from build123d import *

# Parameters (mm, degrees)
ESQUISSE1_R        = 2
BOSS_EXTRU_1_DEPTH = 3


with BuildPart() as part:
    # Esquisse1 → Boss.-Extru.1 (new body)
    with BuildSketch(Plane.XY):
        with BuildLine():
            Line((-5.5, 15), (-25.980762114, 15))
            ThreePointArc((-25.980762114, 15), (-30, 0), (-25.980762114, -15))
            Line((-25.980762114, -15), (25.980762114, -15))
            ThreePointArc((25.980762114, -15), (30, 0), (25.980762114, 15))
            Line((25.980762114, 15), (5.5, 15))
            Line((5.5, 15), (5.5, 4.330127019))
            ThreePointArc((5.5, 4.330127019), (0, -7), (-5.5, 4.330127019))
            Line((-5.5, 4.330127019), (-5.5, 15))
        make_face()
        with Locations((-25, 0)):
            Circle(ESQUISSE1_R, mode=Mode.SUBTRACT)
        with Locations((25, 0)):
            Circle(ESQUISSE1_R, mode=Mode.SUBTRACT)
    extrude(amount=BOSS_EXTRU_1_DEPTH)


solid = part.part
Could you check a few things on this model? Use its own coordinates, in mm. A direction names the side the tool comes from. Give positions to 0.01 mm unless a question says otherwise; leave off trailing zeros. Order: outer loops, then holes, each group sorted by start corner. A loop starts at its lowest first (then second) coordinate and runs counter-clockwise, first axis right, second up.
1. For faces 1 (the flat face through (6, 4, 0)), 2 (the flat face through (5.5, 10, 1)), which set-ups out of +Z, -Z, +X, -X, +Y, -Y let a thin tool reach every point of the face, with its end or its side?
2. Suppose I cut it at B-B (y = 0). List the corners of the cut face in (x, z) for me, plus the area to 3 significant figures.
3. Suppose I cut it at A-A (x = -25). List the corners of the cut face in (y, z) for me, plus the area to 3 significant figures.
4. Will this pin go through, and if not, where does the flat tip stop? P1, Ø0.9, axis at y = 8.5, z = 2, coming from the +X side.
5. I need wall thicknesses on L1, parallel to Y at x = 25, z = 2.4; L2, parallel to X at y = 8.5, z = 1.9; L3, parallel to X at y = -6, z = 1.35. Which ranges of each line are inside material? Lowest first, please.
6. We'd pull the mould along Y, two halves only. Please class faces 3 (the cylindrical face through (-27, 0, 1)), 4 (the flat face through (-16, 15, 1)), 5 (the flat face through (0, -15, 1)), 6 (the cylindrical face through (-30, 0, 1)): pulls with the +Y half, pulls with the -Y half, needs draft (parallel to the pull), parting line crosses it, or undercut.
7. Suppose I cut it at D-D (y = 7.75). List the corners of the cut face in (x, z) for me.
8. Suppose I cut it at C-C (z = 0.9). List the corners of the cut face in (x, y) for me.
Solved:
1. face 1: -Z, +X, -X, +Y, -Y
1. face 2: +Z, -Z, +Y
2. outline: (-30, 0) - (-27, 0) - (-27, 3) - (-30, 3) - close; (-23, 0) - (-7, 0) - (-7, 3) - (-23, 3) - close; (7, 0) - (23, 0) - (23, 3) - (7, 3) - close; (27, 0) - (30, 0) - (30, 3) - (27, 3) - close
2. area: 114 mm2
3. outline: (-15, 0) - (-2, 0) - (-2, 3) - (-15, 3) - close; (2, 0) - (15, 0) - (15, 3) - (2, 3) - close
3. area: 78.0 mm2
4. P1: stops at x = 28.9
5. L1: y = -15 to -2, 2 to 15
5. L2: x = -28.77 to -5.5, 5.5 to 28.77
5. L3: x = -29.39 to -3.61, 3.61 to 29.39
6. face 3: undercut
6. face 4: pulls with the +Y half
6. face 5: pulls with the -Y half
6. face 6: parting line crosses it
7. outline: (-28.98, 0) - (-5.5, 0) - (-5.5, 3) - (-28.98, 3) - close; (5.5, 0) - (28.98, 0) - (28.98, 3) - (5.5, 3) - close
8. outline: (-25.98, -15) - (25.98, -15) arc R30 ccw to (25.98, 15) - (5.5, 15) - (5.5, 4.33) arc R7 cw (long way) to (-5.5, 4.33) - (-5.5, 15) - (-25.98, 15) arc R30 ccw to start; hole circle Ø4 at (-25, 0); hole circle Ø4 at (25, 0)
